from build123d import *

# Parameters (mm, degrees)
F1_DEPTH       = 250
F2_W           = 38
F2_H           = 13
F3_DEPTH       = 250
F4_T1_DEPTH    = 509.3674969976
F5_R           = 9
F6_R           = 1
F8_DEPTH       = 500.001
F10_DEPTH      = 10.482205926
F10_DEPTH_BACK = 13.0380992553
F12_DEPTH      = 13.0380993553
F12_DEPTH_BACK = 10.4822060387
F13_F1_R       = 4.9999
F13_F2_R       = 5
F13_F3_R       = 5
F13_F4_R       = 4.9999
F13_F5_R       = 5
F13_F6_R       = 5


# Not quite as in the source:
# - a fillet or chamfer that OpenCascade refuses, or shapes differently, is made with other operations: its cross-section is extruded or revolved along the edge and cut away or added
# - a fillet or chamfer is up to 0.001 mm smaller than in the source, because OpenCascade refuses the exact size


with BuildPart() as f1:
    # F0 (on Front) → F1 (new body, symmetric)
    with BuildSketch(Plane.XZ):
        with BuildLine():
            Line((22.5, 11.7370992553), (0, 11.7370992553))
            Line((0, 11.7370992553), (-22.5, 11.7370992553))
            Line((-22.5, 11.7370992553), (-22.5, 13.0370992553))
            Line((-22.5, 13.0370992553), (-45.5824640741, 13.0370992553))
            Line((-45.5824640741, 13.0370992553), (-57.5, 3.0370992553))
            Line((-57.5, 3.0370992553), (-57.5, -0.9629007447))
            Line((-57.5, -0.9629007447), (-40.1794919243, -10.9629007447))
            ThreePointArc((-40.1794919243, -10.9629007447), (0, -6.8853558863), (40.1794919243, -10.9629007447))
            Line((40.1794919243, -10.9629007447), (57.5, -0.9629007447))
            Line((57.5, -0.9629007447), (57.5, 3.0370992553))
            Line((57.5, 3.0370992553), (45.5824640741, 13.0370992553))
            Line((45.5824640741, 13.0370992553), (22.5, 13.0370992553))
            Line((22.5, 13.0370992553), (22.5, 11.7370992553))
        make_face()
    extrude(amount=F1_DEPTH, both=True)

    # F2 (on Front) → F3 (cut, symmetric)
    with BuildSketch(Plane.XZ):
        with Locations((0, 3.2370992553)):
            Rectangle(F2_W, F2_H)
    extrude(amount=F3_DEPTH, both=True, mode=Mode.SUBTRACT)

    # F4: fillet of radius 2 on 2 edges, made by hand

    # F4_s2 → F4_t1 (cut)
    with BuildSketch(Plane.XZ.offset(-254.6837484988)):
        with BuildLine():
            ThreePointArc((-22.5, 11.7370992553), (-23.2333239744, 12.6802669278), (-24.3734993995, 13.0370992553))
            Line((-24.3734993995, 13.0370992553), (-22.5, 13.0370992553))
            Line((-22.5, 13.0370992553), (-22.5, 11.7370992553))
        make_face()
        with BuildLine():
            ThreePointArc((24.3734993995, 13.0370992553), (23.2333239744, 12.6802669278), (22.5, 11.7370992553))
            Line((22.5, 11.7370992553), (22.5, 13.0370992553))
            Line((22.5, 13.0370992553), (24.3734993995, 13.0370992553))
        make_face()
    extrude(amount=F4_T1_DEPTH, mode=Mode.SUBTRACT)

    # F5
    f5_edges = [f1.edges().sort_by_distance(p)[0] for p in [
        (-45.582464, 0, 13.037099),
        (45.582464, 0, 13.037099),
        (-40.179492, 0, -10.962901),
        (40.179492, 0, -10.962901),
    ]]
    fillet(f5_edges, radius=F5_R)

    # F6
    f6_edges = [f1.edges().sort_by_distance(p)[0] for p in [
        (57.5, 0, 3.037099),
        (57.5, 0, -0.962901),
        (-57.5, 0, 3.037099),
        (-57.5, 0, -0.962901),
    ]]
    fillet(f6_edges, radius=F6_R)

    # F7 (on face) → F8 (cut, through all)
    with BuildSketch(Plane.XZ.offset(250)):
        with BuildLine():
            ThreePointArc((-42.1022690923, -7.5433837525), (-39.7790673433, -8.3815788055), (-37.3093701274, -8.3607707572))
            ThreePointArc((-37.3093701274, -8.3607707572), (-29.1789785809, -7.0039230093), (-21, -5.9799054874))
            Line((-21, -5.9799054874), (-21, 9.7370992553))
            Line((-21, 9.7370992553), (-22.5, 9.7370992553))
            ThreePointArc((-22.5, 9.7370992553), (-23.2333239744, 10.6802669278), (-24.3734993995, 11.0370992553))
            Line((-24.3734993995, 11.0370992553), (-42.3067319657, 11.0370992553))
            ThreePointArc((-42.3067319657, 11.0370992553), (-44.7008729689, 10.6149476008), (-46.8062452335, 9.3994103571))
            Line((-46.8062452335, 9.3994103571), (-55.7563117574, 1.8894128378))
            ThreePointArc((-55.7563117574, 1.8894128378), (-56.1097188459, 1.036212652), (-55.6135241478, 0.2573429909))
            Line((-55.6135241478, 0.2573429909), (-42.1022690923, -7.5433837525))
        make_face()
        with BuildLine():
            Line((55.7563117574, 1.8894128378), (46.8062452335, 9.3994103571))
            ThreePointArc((46.8062452335, 9.3994103571), (44.7008729689, 10.6149476008), (42.3067319657, 11.0370992553))
            Line((42.3067319657, 11.0370992553), (24.3734993995, 11.0370992553))
            ThreePointArc((24.3734993995, 11.0370992553), (23.2333239744, 10.6802669278), (22.5, 9.7370992553))
            Line((22.5, 9.7370992553), (21, 9.7370992553))
            Line((21, 9.7370992553), (21, -5.9799054874))
            ThreePointArc((21, -5.9799054874), (29.1789785809, -7.0039230093), (37.3093701274, -8.3607707572))
            ThreePointArc((37.3093701274, -8.3607707572), (39.7790673433, -8.3815788055), (42.1022690923, -7.5433837525))
            Line((42.1022690923, -7.5433837525), (55.6135241478, 0.2573429909))
            ThreePointArc((55.6135241478, 0.2573429909), (56.1097188459, 1.036212652), (55.7563117574, 1.8894128378))
        make_face()
    extrude(amount=-F8_DEPTH, mode=Mode.SUBTRACT)

    # F9 (on Top) → F10 (cut, two sides)
    with BuildSketch(Plane.XY) as f10_sk:
        with BuildLine():
            ThreePointArc((-57.5, 200), (0, 257.5), (57.5, 200))
            Line((57.5, 200), (57.5, 280))
            Line((57.5, 280), (-57.5, 280))
            Line((-57.5, 280), (-57.5, 200))
        make_face()
    extrude(amount=-F10_DEPTH, mode=Mode.SUBTRACT)
    extrude(f10_sk.sketch, amount=F10_DEPTH_BACK, mode=Mode.SUBTRACT)

    # F11 (on Top) → F12 (cut, two sides)
    with BuildSketch(Plane.XY) as f12_sk:
        Polygon((16, -140), (-16, -140), (-16, -250), (-43.2975540478, -250), (-68, -216), (-68, -346), (68, -346), (68, -216), (43.2975540478, -250), (16, -250), align=None)
    extrude(amount=F12_DEPTH, mode=Mode.SUBTRACT)
    extrude(f12_sk.sketch, amount=-F12_DEPTH_BACK, mode=Mode.SUBTRACT)

    # F13: fillet of radius 5 on 8 edges, made by hand

    # F13_f1 (radius 5 in the source; OpenCascade refuses exactly that, so slightly less here)
    f13_f1_edges = [f1.edges().sort_by_distance(p)[0] for p in [
        (16, -250, -5.3946419605),
    ]]
    fillet(f13_f1_edges, radius=F13_F1_R)

    # F13_f2
    f13_f2_edges = [f1.edges().sort_by_distance(p)[0] for p in [
        (16, -140, -5.3946419605),
    ]]
    fillet(f13_f2_edges, radius=F13_F2_R)

    # F13_f3
    f13_f3_edges = [f1.edges().sort_by_distance(p)[0] for p in [
        (16, -140, 10.7370992553),
    ]]
    fillet(f13_f3_edges, radius=F13_F3_R)

    # F13_f4 (radius 5 in the source; OpenCascade refuses exactly that, so slightly less here)
    f13_f4_edges = [f1.edges().sort_by_distance(p)[0] for p in [
        (-16, -250, 10.7370992553),
    ]]
    fillet(f13_f4_edges, radius=F13_F4_R)

    # F13_f5
    f13_f5_edges = [f1.edges().sort_by_distance(p)[0] for p in [
        (-16, -140, -5.3946419605),
    ]]
    fillet(f13_f5_edges, radius=F13_F5_R)

    # F13_f6
    f13_f6_edges = [f1.edges().sort_by_distance(p)[0] for p in [
        (-16, -140, 10.7370992553),
    ]]
    fillet(f13_f6_edges, radius=F13_F6_R)


solid = f1.part
Can you work these out from the model? Positions are in its coordinate system, mm. A direction names the side the tool comes from. Coordinates: 2 decimals unless noted, no trailing zeros. Answer as a JSON object with one key per item and string values. Group by question number.
Q1. Imagine slicing it at A-A (y = -170.5). Give the number of separate pieces and of enclosed holes in the cut face, and give its area (3 significant figures).
Q2. I need wall thicknesses on line 1 (Z direction, x = -16, y = -88); line 2 (X direction, y = -52, z = 3); line 3 (Z direction, x = 28.5, y = 86.5). Which ranges of each line are inside material? Lowest first, please. Write a range as from..to.
Q3. Will these pins go through, and if not, where does the flat tip stop? P1, Ø9, axis at x = -29, y = -41.5, coming from the -Z side; P2, Ø0.8, axis at x = 21.5, y = 42.5, coming from the -Z side; P3, Ø22.5, axis at x = 3.5, y = 41.5, coming from the +Z side.
Q4. We'd pull the mould along Z, two halves only. Please class faces 1 (the face through (33, -4, 11.037)), 2 (the face through (49.95, -9.39, -5.32)), 3 (the face through (0, 52, 11.737)): +Z half, -Z half, draft (parallel to the pull), parting line (faces both ways), or undercut.
Q5. On a 3-axis mill with a long thin cutter (end or side, diameter ignored), from which of +Z, -Z, +X, -X, +Y, -Y can I reach the whole of each face in a straight line? I mean faces 4 (the face through (-52.55, -9.27, 7.19)), 5 (the face through (29.065, -3.5, -6.987)). Say none if no direction works.
Determined:
{
 "1": {"separate pieces": "2", "enclosed holes": "2", "area": "434 mm2"},
 "2": {"line 1": "z = -7.53..-3.26, 9.74..11.74", "line 2": "x = -57.4..-54.43, -21..-19, 19..21, 54.43..57.4", "line 3": "z = -8.93..-6.91, 11.04..13.04"},
 "3": {"P1": "stops at z = -9.71", "P2": "stops at z = -8.09", "P3": "stops at z = 11.74"},
 "4": {"face 1": "undercut", "face 2": "-Z half", "face 3": "+Z half"},
 "5": {"face 4": "+Z, -X, +Y, -Y", "face 5": "+Y, -Y"}
}
